For this review, take the finished solid that the model builds, in its own axes (mm). Face numbers are marked on the shaded views. A direction names the side the tool comes from. Give positions to 0.01 mm unless a question says otherwise; leave off trailing zeros. Order: outer loops, then holes, each group sorted by start corner. A loop starts at its lowest first (then second) coordinate and runs counter-clockwise, first axis right, second up. Notation, with made-up numbers: M 9.5,14 L 55.5,14 A15 cw 55.5,28 Z; hole C 62.5,-7.5 d1. An arc over 180 degrees is marked long. Use CSV: the item, a comma, the result in double quotes. Start each with the question number.
(1) Consider section B-B (z = -12). Write out the cut boundary in (x, y).
(2) Draft analysis for pull direction X (two halves, no side actions). For the marked faces 1, 2, 3 and 4, state which applies: pulls with the +X half, pulls with the -X half, needs draft (parallel to the pull), parting line crosses it, or undercut.
(3) Clearance check with flat-ended pins moving along their axes: P1, Ø4, axis at y = -6.5, z = 18.5, coming from the +X side; P2, Ø5, axis at x = 11.5, z = -15, coming from the +Y side; P3, Ø9, axis at y = -21, z = -3, coming from the +X side; P4, Ø4, axis at y = -14.5, z = -14, coming from the +X side. State where each tip first meets the part, or that it passes through.
(4) Consider section A-A (y = -15). Write out the cut boundary in (x, z).
(5) Wall thickness on L1, parallel to X at y = -2.75, z = -12.5; L2, parallel to X at y = -14.25, z = 11; L3, parallel to Z at x = 0, y = -13: over which ranges is each line inside the solid? List them lowest first. Write a range as from..to.
(6) Consider section C-C (x = 0). Write out the cut boundary in (y, z).
(7) Tool access review of the marked faces 5 and 6: name each direction out of +Z, -Z, +X, -X, +Y, -Y from which nothing blocks a thin tool from reaching the whole face with its end or side.
```python
from build123d import *

# Parameters (mm, degrees)
F1_DEPTH  = 30
F2_R      = 10
F3_DEPTH  = 30.001
F5_DEPTH  = 30.001
F7_DEPTH  = 2
F8_R      = 4
F9_DEPTH  = 5
F10_SIZE2 = 2
F10_SIZE  = 2


with BuildPart() as f1:
    # F0 (on Front) → F1 (new body)
    with BuildSketch(Plane.XZ):
        with BuildLine():
            Line((-14.9850390488, 11.2684052181), (-14.9850390488, -24.4013743764))
            Line((-14.9850390488, -24.4013743764), (-0.9850390488, -24.4013743764))
            Line((-0.9850390488, -24.4013743764), (1, -24.4013743764))
            Line((1, -24.4013743764), (15, -24.4013743764))
            Line((15, -24.4013743764), (15, 10.5986256236))
            ThreePointArc((15, 10.5986256236), (0.334973333, 25.5948849194), (-14.9850390488, 11.2684052181))
        make_face()
    extrude(amount=F1_DEPTH)

    # F2 (on face) → F3 (cut, through all)
    with BuildSketch(Plane.XZ.offset(30)):
        with Locations((0, 10.5986256236)):
            Circle(F2_R)
    extrude(amount=-F3_DEPTH, mode=Mode.SUBTRACT)

    # F4 (on face) → F5 (cut, through all)
    with BuildSketch(Plane.XZ.offset(30)):
        with BuildLine():
            Line((-1, -24.4013743764), (0, -24.4013743764))
            Line((0, -24.4013743764), (1, -24.4013743764))
            Line((1, -24.4013743764), (1, 0.6487512526))
            ThreePointArc((1, 0.6487512526), (0, 0.5986256236), (-1, 0.6487512526))
            Line((-1, 0.6487512526), (-1, -24.4013743764))
        make_face()
    extrude(amount=-F5_DEPTH, mode=Mode.SUBTRACT)

    # F6 (on face) → F7 (cut)
    with BuildSketch(Plane.YZ.offset(15)):
        with BuildLine():
            Line((0, -24.4013743764), (0, -1.172617821))
            ThreePointArc((0, -1.172617821), (-15, 5.5986256236), (-30, -1.172617821))
            Line((-30, -1.172617821), (-30, -24.4013743764))
            Line((-30, -24.4013743764), (0, -24.4013743764))
        make_face()
    extrude(amount=-F7_DEPTH, mode=Mode.SUBTRACT)

    # F8 (on face) → F9 (cut, symmetric)
    with BuildSketch(Plane.YZ.offset(13)):
        with Locations((-15, -14.4013743764)):
            Circle(F8_R)
    extrude(amount=F9_DEPTH, both=True, mode=Mode.SUBTRACT)

    # F10
    f10_edges = [f1.edges().sort_by_distance(p)[0] for p in [
        (0, -30, 20.598626),
        (0, 0, 20.598626),
    ]]
    chamfer(f10_edges, length=F10_SIZE, length2=F10_SIZE2)


solid = f1.part
```
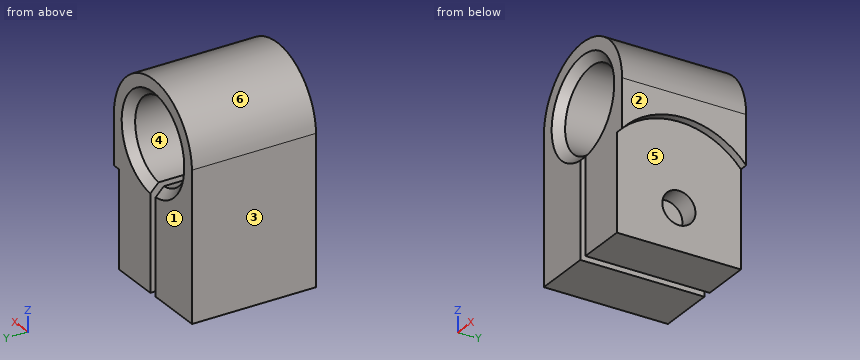
Check result:
1,outline,"M -14.99,-30 L -1,-30 L -1,0 L -14.99,0 Z; M 1,-30 L 13,-30 L 13,-18.2 L 8,-18.2 L 8,-11.8 L 13,-11.8 L 13,0 L 1,0 Z"
2,face 1,"needs draft"
2,face 2,"pulls with the +X half"
2,face 3,"pulls with the -X half"
2,face 4,"undercut"
3,P1,"stops at x = 13.79"
3,P2,"stops at y = 0"
3,P3,"stops at x = 13"
3,P4,"stops at x = 8"
4,outline,"M -14.99,-24.4 L -1,-24.4 L -1,0.65 A10 cw long 1,0.65 L 1,-24.4 L 13,-24.4 L 13,-18.4 L 8,-18.4 L 8,-10.4 L 13,-10.4 L 13,5.6 L 15,5.6 L 15,10.6 A15 ccw -14.99,11.27 Z"
5,L1,"x = -14.99..-1, 1..13"
5,L2,"x = -14.99..-9.99, 9.99..14.99"
5,L3,"z = 20.6..25.6"
6,outline,"M -30,22.6 L -28,20.6 L -2,20.6 L 0,22.6 L 0,25.6 L -30,25.6 Z"
7,face 5,"-Z, +X"
7,face 6,"+Z, +Y, -Y"
